Part model, mm, in its own coordinate system. A direction names the side the tool comes from. Coordinates: 2 decimals unless noted, no trailing zeros. Order: outer loops, then holes, each group sorted by start corner. A loop starts at its lowest first (then second) coordinate and runs counter-clockwise, first axis right, second up.
from build123d import *

# Parameters (mm, degrees)
SKETCH1_W                   = 63.5
SKETCH1_H                   = 12.7
BOSS_EXTRUDE1_DEPTH         = 53.975
CUT_EXTRUDE1_REACH          = 14.7
SKETCH2_W                   = 19.05
SKETCH2_H                   = 95.25
SKETCH3_R                   = 3.302
CUT_EXTRUDE2_DEPTH          = 13.7
F_1_4_20_TAPPED_HOLE1_D     = 5.1054
F_1_4_20_TAPPED_HOLE1_DEPTH = 19.05
F_1_4_20_TAPPED_HOLE1_TIP   = 1.533816902
SKETCH6_W                   = 38.1
SKETCH6_H                   = 2.54
CUT_EXTRUDE3_DEPTH          = 13.7
F_1_4_20_TAPPED_HOLE2_D     = 5.1054
F_1_4_20_TAPPED_HOLE2_DEPTH = 25.4
F_1_4_20_TAPPED_HOLE2_TIP   = 1.533816902


with BuildPart() as part:
    # Sketch1 → Boss-Extrude1 (new body, symmetric)
    with BuildSketch(Plane(origin=(0, 0, 0), x_dir=(1, 0, 0), z_dir=(0, 1, 0))):
        Rectangle(SKETCH1_W, SKETCH1_H)
    extrude(amount=BOSS_EXTRUDE1_DEPTH, both=True)

    # Sketch2 → Cut-Extrude1 (cut, up to next)
    with BuildSketch(Plane.XY.offset(6.35), mode=Mode.PRIVATE) as cut_extrude1_sk1:
        with Locations((-22.225, 6.35)):
            Rectangle(SKETCH2_W, SKETCH2_H)
    cut_extrude1_tool1 = extrude(cut_extrude1_sk1.sketch, amount=-CUT_EXTRUDE1_REACH, mode=Mode.PRIVATE) & part.part
    add(cut_extrude1_tool1.solids().sort_by_distance((-22.225, 6.35, 6.35))[0], mode=Mode.SUBTRACT)
    # Sketch2 → Cut-Extrude1 (cut, up to next)
    with BuildSketch(Plane.XY.offset(6.35), mode=Mode.PRIVATE) as cut_extrude1_sk2:
        with Locations((22.225, 6.35)):
            Rectangle(SKETCH2_W, SKETCH2_H)
    cut_extrude1_tool2 = extrude(cut_extrude1_sk2.sketch, amount=-CUT_EXTRUDE1_REACH, mode=Mode.PRIVATE) & part.part
    add(cut_extrude1_tool2.solids().sort_by_distance((22.225, 6.35, 6.35))[0], mode=Mode.SUBTRACT)

    # Sketch3 → Cut-Extrude2 (cut, through all)
    with BuildSketch(Plane(origin=(0, -41.275, 0), x_dir=(1, 0, 0), z_dir=(0, 1, 0))):
        with Locations((-25.4, 0)):
            Circle(SKETCH3_R)
        with Locations((25.4, 0)):
            Circle(SKETCH3_R)
    extrude(amount=-CUT_EXTRUDE2_DEPTH, mode=Mode.SUBTRACT)

    # 1/4-20 Tapped Hole1
    with Locations(Plane(origin=(0, 53.975, 0), x_dir=(1, 0, 0), z_dir=(0, 1, 0))):
        with Locations((0, 0)):
            Hole(F_1_4_20_TAPPED_HOLE1_D / 2, depth=F_1_4_20_TAPPED_HOLE1_DEPTH)
            with Locations((0, 0, -(F_1_4_20_TAPPED_HOLE1_DEPTH + F_1_4_20_TAPPED_HOLE1_TIP / 2))):  # 118° drill point
                Cone(0, F_1_4_20_TAPPED_HOLE1_D / 2, F_1_4_20_TAPPED_HOLE1_TIP, mode=Mode.SUBTRACT)

    # Sketch6 → Cut-Extrude3 (cut, through all)
    with BuildSketch(Plane.XY.offset(6.35)):
        with Locations((0, -52.705)):
            Rectangle(SKETCH6_W, SKETCH6_H)
    extrude(amount=-CUT_EXTRUDE3_DEPTH, mode=Mode.SUBTRACT)

    # 1/4-20 Tapped Hole2
    with Locations(Plane.XY.offset(6.35)):
        with Locations((0, 15.875)):
            Hole(F_1_4_20_TAPPED_HOLE2_D / 2, depth=F_1_4_20_TAPPED_HOLE2_DEPTH)
            with Locations((0, 0, -(F_1_4_20_TAPPED_HOLE2_DEPTH + F_1_4_20_TAPPED_HOLE2_TIP / 2))):  # 118° drill point
                Cone(0, F_1_4_20_TAPPED_HOLE2_D / 2, F_1_4_20_TAPPED_HOLE2_TIP, mode=Mode.SUBTRACT)


solid = part.part
Q1. Mould opens along X. For faces 6 (the face through (22.1, -47.5, -0.1)), 7 (the face through (-31.75, -48, 0)), 8 (the face through (-22, -41.275, 2)) say: pulls with the +X half, pulls with the -X half, needs draft (parallel to the pull), parting line crosses it, or undercut.
Results list:
face 6: undercut
face 7: pulls with the -X half
face 8: needs draft
Q2. Cut at A-A on x = 25.4. Write the cut outline in (y, z) (3 decimals).
Results list:
outline: (-53.975, -6.35) - (-41.275, -6.35) - (-41.275, -3.302) - (-53.975, -3.302) - close; (-53.975, 3.302) - (-41.275, 3.302) - (-41.275, 6.35) - (-53.975, 6.35) - close
Q3. Wall check: line 1 along X through (y, z) = (-44, 0); line 2 along Z through (x, y) = (25.4, -51); line 3 along Z through (x, y) = (0, 48). Give the ranges that are in metal, low to high.
Results list:
line 1: x = -31.75 to -28.7, -22.1 to 22.1, 28.7 to 31.75
line 2: z = -6.35 to -3.3, 3.3 to 6.35
line 3: z = -6.35 to -2.55, 2.55 to 6.35
Q4. Which spindle directions (+Z, -Z, +X, -X, +Y, -Y) get a long thin tool onto all of the face, cutting with end or side? Do faces 1 (the face through (-19.05, -53, 0)), 2 (the face through (-12.7, 6, 0)), 3 (the face through (31.75, -48, 0)), 4 (the face through (-2.435, 44.317, -0.767)), 5 (the face through (12.7, 6, 0)). Say none if no direction does.
Results list:
face 1: +Z, -Z, -Y
face 2: +Z, -Z, -X, +Y
face 3: +Z, -Z, +X, +Y, -Y
face 4: +Y
face 5: +Z, -Z, +X, +Y
Q5. Pin check, flat tips, straight feed: pin 1 Ø4 at (x, z) = (-14, 5) entering from -Y (3 decimals); pin 2 Ø4 at (x, z) = (-14, -1) entering from +Y (3 decimals); pin 3 Ø6.5 at (x, z) = (-24.5, -2.5) entering from +Y (3 decimals); pin 4 Ø4 at (x, z) = (25.4, 0) entering from -Y. Stop position of each tip, or through.
Results list:
pin 1: stops at y = -51.435
pin 2: stops at y = 53.975
pin 3: stops at y = -41.275
pin 4: passes through
Q6. Cut at D-D on x = -11.5. Write the cut outline in (y, z) (3 decimals), and give its area (3 significant figures).
Results list:
outline: (-51.435, -6.35) - (53.975, -6.35) - (53.975, 6.35) - (-51.435, 6.35) - close
area: 1,340 mm2
Q7. Cut at C-C on z = -5.25. Write the cut outline in (x, y) (3 decimals).
Results list:
outline: (-31.75, -53.975) - (-19.05, -53.975) - (-19.05, -51.435) - (19.05, -51.435) - (19.05, -53.975) - (31.75, -53.975) - (31.75, -41.275) - (12.7, -41.275) - (12.7, 53.975) - (-12.7, 53.975) - (-12.7, -41.275) - (-31.75, -41.275) - close; hole circle Ø5.105 at (0, 15.875)
Q8. Cut at B-B on y = 38. Write the cut outline in (x, z), and give its area (3 significant figures).
Results list:
outline: (-12.7, -6.35) - (12.7, -6.35) - (12.7, 6.35) - (-12.7, 6.35) - close; hole circle Ø5.11 at (0, 0)
area: 302 mm2
